Could you check a few things on this model? Use its own coordinates, in mm. A direction names the side the tool comes from. Give positions to 0.01 mm unless a question says otherwise; leave off trailing zeros. Loops run counter-clockwise (first coordinate to the right, second up) from the corner with the lowest first, then second, coordinate; pieces in that order, holes last. Notation, with made-up numbers: (20.5, -18) - (57.5, -18) arc R26 ccw to (57.5, 14) - close; hole circle Ø2 at (88.25, 80). An arc over 180 degrees is marked (long way). Write each question's results on one line, items separated by ' | '. Start each with the question number.
1) On a 3-axis mill with a long thin cutter (end or side, diameter ignored), from which of +Z, -Z, +X, -X, +Y, -Y can I reach the whole of each face in a straight line? I mean faces 4 (the face through (-6.466, 2.681, 12.374)), 5 (the face through (5, 13, -5)), 6 (the face through (0, 15, -5)), 7 (the face through (0, 10.3, -5)). Say none if no direction works.
2) If we mould it in two halves opening along X, with no side actions, what happens to faces 1 (the face through (-0.2, 7.3, 3.5)), 2 (the face through (14, -13, 2)), 3 (the face through (-5, 13, -5))? For each: +X half, -X half, draft (parallel to the pull), parting line (faces both ways), or undercut.
3) I want a section at B-B, the plane y = 11.5. Write out the boundary of the cut face in (x, z), and give its area (3 significant figures).
4) I want a section at A-A, the plane y = -14. Write out the boundary of the cut face in (x, z), and give its area (3 significant figures).
5) I'm going to push flat-ended pins straight in: pin 1 (1.8 mm diameter, centred on x = 14, y = 14, fed in from -Z); pin 2 (3 mm diameter, centred on y = -0.5, z = 17.5, fed in from -X); pin 3 (1 mm diameter, centred on x = -9.5, y = -11, fed in from +Z); pin 4 (10 mm diameter, centred on x = 1.5, y = -2, fed in from -Z). Where does each tip first touch, or does it pass through?
6) I want a section at C-C, the plane x = 3.5. Write out the boundary of the cut face in (y, z), and give its area (3 significant figures).
7) If I drill on probe 1 along Y at (x, z) = (14, 1.7); probe 2 along Z at (x, y) = (-8.5, -8), over which ranges is the centre line in solid material (lowest first)? Write a range as [from, to].
8) I want a section at D-D, the plane z = -2. Write out the boundary of the cut face in (x, y).
from build123d import *

# Parameters (mm, degrees)
SKETCH1_W           = 32
SKETCH1_H           = 32
BOSS_EXTRUDE1_DEPTH = 3.5
BOSS_EXTRUDE2_START = 3.5
SKETCH2_R           = 7
BOSS_EXTRUDE2_DEPTH = 18
SKETCH3_W           = 10
SKETCH3_H           = 4.7
BOSS_EXTRUDE3_DEPTH = 10
SKETCH4_R           = 1
CUT_EXTRUDE1_DEPTH  = 10


with BuildPart() as part:
    # Sketch1 → Boss-Extrude1 (new body)
    with BuildSketch(Plane.XY):
        Rectangle(SKETCH1_W, SKETCH1_H)
    extrude(amount=BOSS_EXTRUDE1_DEPTH)

    # Sketch2 → Boss-Extrude2 (add)
    with BuildSketch(Plane.XY.offset(BOSS_EXTRUDE2_START)):
        with Locations(Location((0, 0, 0), (0, 0, 180))):
            Circle(SKETCH2_R)
    extrude(amount=BOSS_EXTRUDE2_DEPTH)

    # Sketch3 → Boss-Extrude3 (add)
    with BuildSketch(Plane.XY):
        with Locations((0, 12.65)):
            Rectangle(SKETCH3_W, SKETCH3_H)
    extrude(amount=-BOSS_EXTRUDE3_DEPTH)

    # Sketch4 → Cut-Extrude1 (cut)
    with BuildSketch(Plane.XY):
        with Locations(Location((14, 14, 0), (0, 0, 180))):
            Circle(SKETCH4_R)
        with Locations(Location((-14, 14, 0), (0, 0, 180))):
            Circle(SKETCH4_R)
        with Locations(Location((-14, -14, 0), (0, 0, 180))):
            Circle(SKETCH4_R)
        with Locations(Location((14, -14, 0), (0, 0, 180))):
            Circle(SKETCH4_R)
    extrude(amount=CUT_EXTRUDE1_DEPTH, mode=Mode.SUBTRACT)


solid = part.part
Answers:
1) face 4: +Z | face 5: -Z, +X, +Y, -Y | face 6: -Z, +X, -X, +Y | face 7: -Z, +X, -X, -Y
2) face 1: draft | face 2: undercut | face 3: -X half
3) outline: (-16, 0) - (-5, 0) - (-5, -10) - (5, -10) - (5, 0) - (16, 0) - (16, 3.5) - (-16, 3.5) - close | area: 212 mm2
4) outline: (-16, 0) - (-15, 0) - (-15, 3.5) - (-16, 3.5) - close; (-13, 0) - (13, 0) - (13, 3.5) - (-13, 3.5) - close; (15, 0) - (16, 0) - (16, 3.5) - (15, 3.5) - close | area: 98.0 mm2
5) pin 1: passes through | pin 2: stops at x = -7 | pin 3: stops at z = 3.5 | pin 4: stops at z = 0
6) outline: (-16, 0) - (10.3, 0) - (10.3, -10) - (15, -10) - (15, 0) - (16, 0) - (16, 3.5) - (6.06, 3.5) - (6.06, 21.5) - (-6.06, 21.5) - (-6.06, 3.5) - (-16, 3.5) - close | area: 377 mm2
7) probe 1: y = [-16, -15], [-13, 13], [15, 16] | probe 2: z = [0, 3.5]
8) outline: (-5, 10.3) - (5, 10.3) - (5, 15) - (-5, 15) - close
